Check sheet for the modelled part. Datum: model origin and axes. Units: mm. A direction names the side the tool comes from. Round coordinates to 2 decimals unless told otherwise and drop trailing zeros. Order: outer loops, then holes, each group sorted by start corner. A loop starts at its lowest first (then second) coordinate and runs counter-clockwise, first axis right, second up. Notation, with made-up numbers: M 11,-3 L 34,-3 A24 cw 34,36 Z; hole C 70.25,-30 d2. An arc over 180 degrees is marked long. One line per item, written item: value. Start each with the question number.
(1) Cross-section at A-A, the plane z = 2.55. Enter the section's corners in (x, y) (3 decimals), and give its area (3 significant figures).
(2) Access from +Z, -Z, +X, -X, +Y, -Y to the whole of each face (thin tool, end or side, straight path). Record for faces 4 (the face through (-1.08, -4.88, 1.7)), 5 (the face through (0, 0, 4.9)).
(3) Release check for a two-part mould opening along Y. For faces 1 (the face through (3.84, 1.21, 3.13)), 2 (the face through (5, -2, 0)), 3 (the face through (-0.82, 0.26, 3.45)) record: released by +Y, released by -Y, zero draft, split by the parting line, or undercut.
(4) Thickness scan on L1, parallel to Z at x = -5.25, y = 4.5; L2, parallel to X at y = 1.25, z = 0.7; L3, parallel to Y at x = -0.5, z = 2.45. Record the ranges inside material, lowest first.
(5) Depth check by flat-ended pin: pin 1 Ø5 at (x, y) = (-3, 1) entering from -Z; pin 2 Ø1.5 at (x, z) = (-0.5, 3.5) entering from +Y (3 decimals). Enter the tip coordinate at first touch or a pass-through.
from build123d import *

# Parameters (mm, degrees)
F0_R     = 8
F1_DEPTH = 1.5
F2_R     = 5
F3_DEPTH = 0.4
F4_R     = 4.025
F5_DEPTH = 3
F6_SIZE  = 0.5


with BuildPart() as f1:
    # F0 (on Top) → F1 (new body)
    with BuildSketch(Plane.XY):
        Circle(F0_R)
    extrude(amount=F1_DEPTH)

    # F2 (on face) → F3 (join)
    with BuildSketch(Plane.XY.offset(1.5)):
        Circle(F2_R)
    extrude(amount=F3_DEPTH)

    # F4 (on face) → F5 (join)
    with BuildSketch(Plane.XY.offset(1.9)):
        Circle(F4_R)
    extrude(amount=F5_DEPTH)

    # F6
    f6_edges = [f1.edges().sort_by_distance(p)[0] for p in [
        (-8, 0, 0),
        (-8, 0, 1.5),
        (-4.025, 0, 4.9),
    ]]
    chamfer(f6_edges, length=F6_SIZE)

    # F7 (on Front) → F8 (revolve, cut)
    with BuildSketch(Plane.XZ):
        Polygon((0, 4.170951), (-4.970746, 0), (0, 0), align=None)
    revolve(axis=Axis((0, 0, 2.085476), (0, 0, -1)), mode=Mode.SUBTRACT)


solid = f1.part
Values found:
1. outline: C 0,0 d8.05; hole C 0,0 d3.864
1. area: 39.2 mm^2
2. face 4: +Z
2. face 5: +Z, +X, -X, +Y, -Y
3. face 1: split by the parting line
3. face 2: zero draft
3. face 3: undercut
4. L1: 0 to 1.5
4. L2: -7.9 to -3.94, 3.94 to 7.9
4. L3: -3.99 to -1.99, 1.99 to 3.99
5. pin 1: z = 0
5. pin 2: y = 4.025
